Can you work these out from the model? Positions are in its coordinate system, mm. A direction names the side the tool comes from. Give positions to 0.01 mm unless a question says otherwise; leave off trailing zeros. Order: outer loops, then holes, each group sorted by start corner. A loop starts at its lowest first (then second) coordinate and runs counter-clockwise, first axis right, second up. Notation, with made-up numbers: (87, 10) - (110, 10) arc R21 ccw to (110, 17) - close; hole circle Ø3 at (44.5, -36). An arc over 180 degrees is marked (long way). Use one line per item in the form item = value. Start each with the question number.
1) For pin 1 (3 mm diameter, centred on x = 4.5, z = 6, fed in from +Y); pin 2 (2 mm diameter, centred on x = 0.5, z = 1, fed in from +Y); pin 3 (8 mm diameter, centred on y = -20.5, z = 6, fed in from +X); pin 4 (2 mm diameter, centred on x = 26.25, y = -24.5, fed in from -Z), each with a flat end and sliding along its axis, tell me the tip position at first contact or that it passes through.
2) We'd pull the mould along Y, two halves only. Please class faces 1 (the flat face through (30.5, 0, 14)), 2 (the cylindrical face through (0, -19, 1)), 3 (the cylindrical face through (7.76, -25.26, 13.77)): released by +Y, released by -Y, zero draft, split by the parting line, or undercut.
3) Which directions (+Z, -Z, +X, -X, +Y, -Y) give clear straight access to the entire face, cutting with the end or side of a thin tool? Please do faces 4 (the flat face through (0, 19, 15)), 5 (the cylindrical face through (0, 17, 3)), 6 (the flat face through (21.5, 0, 7)).
4) Suppose I cut it at B-B, the plane y = 24.5. Write out the boundary of the cut face in (x, z), and give its area (4 significant figures).
5) Suppose I cut it at D-D, the plane z = 6.25. Write out the boundary of the cut face in (x, y), and give its area (3 significant figures).
6) Please list where these lines run through material, in increasing order: probe 1 along Y at (x, z) = (26.25, 13.7); probe 2 along Y at (x, z) = (-8.75, 13.9); probe 3 along X at (y, z) = (-5, 11.5).
7) Suppose I cut it at C-C, the plane x = 8.75. Write out the boundary of the cut face in (y, z).
8) Suppose I cut it at A-A, the plane x = -26.25. Write out the boundary of the cut face in (y, z).
```python
from build123d import *

# Parameters (mm, degrees)
SKETCH1_W           = 43
SKETCH1_H           = 39
BOSS_EXTRUDE1_DEPTH = 12.5
SHELL1_T            = -2
SKETCH2_W           = 61
SKETCH2_H           = 57
SKETCH2_W_2         = 39
SKETCH2_H_2         = 35
BOSS_EXTRUDE2_DEPTH = 2.5
FILLET1_R           = 2.5
FILLET2_R           = 2.5
SKETCH3_W           = 15
SKETCH3_H           = 8
CUT_EXTRUDE1_DEPTH  = 44.720704477
SKETCH4_R           = 1.25
CUT_EXTRUDE2_DEPTH  = 2.5


with BuildPart() as part:
    # Sketch1 → Boss-Extrude1 (new body)
    with BuildSketch(Plane.XY):
        Rectangle(SKETCH1_W, SKETCH1_H)
    extrude(amount=BOSS_EXTRUDE1_DEPTH)

    # Shell1
    shell1_openings = [part.faces().sort_by_distance(p)[0] for p in [
        (0, 0, 12.5),
    ]]
    offset(amount=SHELL1_T, openings=shell1_openings, kind=Kind.INTERSECTION)

    # Sketch2 → Boss-Extrude2 (add)
    with BuildSketch(Plane.XY.offset(12.5)):
        Rectangle(SKETCH2_W, SKETCH2_H)
        Rectangle(SKETCH2_W_2, SKETCH2_H_2, mode=Mode.SUBTRACT)
    extrude(amount=BOSS_EXTRUDE2_DEPTH)

    # Fillet1
    fillet1_edges = [part.edges().sort_by_distance(p)[0] for p in [
        (30.5, -28.5, 13.75),
        (30.5, 28.5, 13.75),
        (-30.5, 28.5, 13.75),
        (-30.5, -28.5, 13.75),
    ]]
    fillet(fillet1_edges, radius=FILLET1_R)

    # Fillet2
    fillet2_edges = [part.edges().sort_by_distance(p)[0] for p in [
        (19.5, 0, 2),
        (0, 17.5, 2),
        (-19.5, 0, 2),
        (0, -17.5, 2),
        (0, -19.5, 0),
        (-21.5, 0, 0),
        (0, 19.5, 0),
        (21.5, 0, 0),
        (21.5, -19.5, 6.25),
        (-21.5, -19.5, 6.25),
        (-21.5, 19.5, 6.25),
        (21.5, 19.5, 6.25),
    ]]
    fillet(fillet2_edges, radius=FILLET2_R)

    # Sketch3 → Cut-Extrude1 (cut, through all)
    with BuildSketch(Plane.XY.offset(2)):
        with Locations((0, 10)):
            Rectangle(SKETCH3_W, SKETCH3_H)
    extrude(amount=-CUT_EXTRUDE1_DEPTH, mode=Mode.SUBTRACT)

    # Sketch4 → Cut-Extrude2 (cut)
    with BuildSketch(Plane.XY.offset(15)):
        with Locations((-26.25, 24.5)):
            Circle(SKETCH4_R)
        with Locations((-8.75, 24.5)):
            Circle(SKETCH4_R)
        with Locations((8.75, 24.5)):
            Circle(SKETCH4_R)
        with Locations((26.25, 24.5)):
            Circle(SKETCH4_R)
        with Locations((26.25, 8.166666667)):
            Circle(SKETCH4_R)
        with Locations((26.25, -8.166666667)):
            Circle(SKETCH4_R)
        with Locations((-8.75, -24.5)):
            Circle(SKETCH4_R)
        with Locations((8.75, -24.5)):
            Circle(SKETCH4_R)
        with Locations((26.25, -24.5)):
            Circle(SKETCH4_R)
        with Locations((-26.25, 8.166666667)):
            Circle(SKETCH4_R)
        with Locations((-26.25, -8.166666667)):
            Circle(SKETCH4_R)
        with Locations((-26.25, -24.5)):
            Circle(SKETCH4_R)
    extrude(amount=-CUT_EXTRUDE2_DEPTH, mode=Mode.SUBTRACT)


solid = part.part
```
Result sheet:
q1.pin_1 = 19.5
q1.pin_2 = 19.45
q1.pin_3 = 21.5
q1.pin_4 = through
q2.face_1 = zero draft
q2.face_2 = released by -Y
q2.face_3 = undercut
q3.face_4 = +Z, +X, -X, +Y, -Y
q3.face_5 = +Z
q3.face_6 = -Z, +X, +Y, -Y
q4.outline = (-30.5, 12.5) - (-27.5, 12.5) - (-27.5, 15) - (-30.5, 15) - close; (-25, 12.5) - (-10, 12.5) - (-10, 15) - (-25, 15) - close; (-7.5, 12.5) - (7.5, 12.5) - (7.5, 15) - (-7.5, 15) - close; (10, 12.5) - (25, 12.5) - (25, 15) - (10, 15) - close; (27.5, 12.5) - (30.5, 12.5) - (30.5, 15) - (27.5, 15) - close
q4.area = 127.5 mm²
q5.outline = (-21.5, -17) arc R2.5 ccw to (-19, -19.5) - (19, -19.5) arc R2.5 ccw to (21.5, -17) - (21.5, 17) arc R2.5 ccw to (19, 19.5) - (-19, 19.5) arc R2.5 ccw to (-21.5, 17) - close; hole (-19.5, -17.5) - (19.5, -17.5) - (19.5, 17.5) - (-19.5, 17.5) - close
q5.area = 307 mm²
q6.probe_1 = -28.5 to -25.75, -23.25 to -9.42, -6.92 to 6.92, 9.42 to 23.25, 25.75 to 28.5
q6.probe_2 = -28.5 to -25.75, -23.25 to -17.5, 17.5 to 23.25, 25.75 to 28.5
q6.probe_3 = -21.5 to -19.5, 19.5 to 21.5
q7.outline = (-28.5, 12.5) - (-25.75, 12.5) - (-25.75, 15) - (-28.5, 15) - close; (-23.25, 12.5) - (-19.5, 12.5) - (-19.5, 2.5) arc R2.5 ccw to (-17, 0) - (17, 0) arc R2.5 ccw to (19.5, 2.5) - (19.5, 12.5) - (23.25, 12.5) - (23.25, 15) - (17.5, 15) - (17.5, 4.5) arc R2.5 cw to (15, 2) - (-15, 2) arc R2.5 cw to (-17.5, 4.5) - (-17.5, 15) - (-23.25, 15) - close; (25.75, 12.5) - (28.5, 12.5) - (28.5, 15) - (25.75, 15) - close
q8.outline = (-28.5, 12.5) - (-25.75, 12.5) - (-25.75, 15) - (-28.5, 15) - close; (-23.25, 12.5) - (-9.42, 12.5) - (-9.42, 15) - (-23.25, 15) - close; (-6.92, 12.5) - (6.92, 12.5) - (6.92, 15) - (-6.92, 15) - close; (9.42, 12.5) - (23.25, 12.5) - (23.25, 15) - (9.42, 15) - close; (25.75, 12.5) - (28.5, 12.5) - (28.5, 15) - (25.75, 15) - close
